```python
from build123d import *

# Parameters (mm, degrees)
SKETCH_1_W                     = 86.9
SKETCH_1_H                     = 86.9
EXTRUDE_1_DEPTH                = 3
HOLE_WIZARD_M2_5_1_D           = 3
HOLE_WIZARD_M2_5_1_DEPTH       = 3
HOLE_WIZARD_M2_5_1_CBORE_D     = 6
HOLE_WIZARD_M2_5_1_CBORE_DEPTH = 2
HOLE_WIZARD_2_0_2_1_D          = 2
HOLE_WIZARD_2_0_2_1_DEPTH      = 3
HOLE_WIZARD_2_5_2_5_1_D        = 2.5
HOLE_WIZARD_2_5_2_5_1_DEPTH    = 3
FILLET_1_R                     = 3
SKETCH_8_R                     = 14
CUT_EXTRUDE_1_DEPTH            = 4


with BuildPart() as part:
    # 草圖1 → 填料-伸長1 (new body)
    with BuildSketch(Plane(origin=(0, -37, 0), x_dir=(1, 0, 0), z_dir=(0, 1, 0))):
        Rectangle(SKETCH_1_W, SKETCH_1_H)
    extrude(amount=-EXTRUDE_1_DEPTH)

    # M2.5 六角頭機械螺釘的柱孔1
    with Locations(Plane(origin=(0, -40, 0), x_dir=(-1, 0, 0), z_dir=(0, -1, 0))):
        with Locations((39, 39), (-39, 39), (-39, -39), (39, -39)):
            CounterBoreHole(HOLE_WIZARD_M2_5_1_D / 2, HOLE_WIZARD_M2_5_1_CBORE_D / 2, HOLE_WIZARD_M2_5_1_CBORE_DEPTH, depth=HOLE_WIZARD_M2_5_1_DEPTH)

    # Ø2.0 (2) 直徑孔1
    with Locations(Plane(origin=(0, -37, 0), x_dir=(1, 0, 0), z_dir=(0, 1, 0))):
        with Locations((5, -10), (0, -10), (-5, -10), (-10, -5), (-10, 0), (-10, 5), (-5, 10), (0, 10), (5, 10), (10, 5), (10, 0), (10, -5), (5, -5), (0, -5), (-5, -5), (-5, 0), (-5, 5), (0, 5), (5, 5), (5, 0), (0, 0), (-37.5, 3), (-37.5, 0), (-37.5, -3), (3, 37.5), (0, 37.5), (-3, 37.5), (37.5, -3), (37.5, 0), (37.5, 3), (-3, -37.5), (0, -37.5), (3, -37.5)):
            Hole(HOLE_WIZARD_2_0_2_1_D / 2, depth=HOLE_WIZARD_2_0_2_1_DEPTH)

    # Ø2.5 (2.5) 直徑孔1
    with Locations(Plane(origin=(0, -40, 0), x_dir=(-1, 0, 0), z_dir=(0, -1, 0))):
        with Locations((12, 12), (-12, 12), (12, -12), (-12, -12)):
            Hole(HOLE_WIZARD_2_5_2_5_1_D / 2, depth=HOLE_WIZARD_2_5_2_5_1_DEPTH)

    # 圓角1
    fillet_1_edges = [part.edges().sort_by_distance(p)[0] for p in [
        (-43.45, -38.5, -43.45),
        (43.45, -38.5, -43.45),
        (43.45, -38.5, 43.45),
        (-43.45, -38.5, 43.45),
    ]]
    fillet(fillet_1_edges, radius=FILLET_1_R)

    # 草圖8 → 除料-伸長1 (cut, through all)
    with BuildSketch(Plane(origin=(0, -37, 0), x_dir=(1, 0, 0), z_dir=(0, 1, 0))):
        Circle(SKETCH_8_R)
        with BuildLine():
            Line((-40.45, -12), (-40.45, 12))
            ThreePointArc((-40.45, 12), (-37.45, 15), (-34.45, 12))
            Line((-34.45, 12), (-34.45, -12))
            ThreePointArc((-34.45, -12), (-37.45, -15), (-40.45, -12))
        make_face()
        with BuildLine():
            Line((-12, 40.45), (12, 40.45))
            ThreePointArc((12, 40.45), (15, 37.45), (12, 34.45))
            Line((12, 34.45), (-12, 34.45))
            ThreePointArc((-12, 34.45), (-15, 37.45), (-12, 40.45))
        make_face()
        with BuildLine():
            Line((40.45, 12), (40.45, -12))
            ThreePointArc((40.45, -12), (37.45, -15), (34.45, -12))
            Line((34.45, -12), (34.45, 12))
            ThreePointArc((34.45, 12), (37.45, 15), (40.45, 12))
        make_face()
        with BuildLine():
            Line((12, -40.45), (-12, -40.45))
            ThreePointArc((-12, -40.45), (-15, -37.45), (-12, -34.45))
            Line((-12, -34.45), (12, -34.45))
            ThreePointArc((12, -34.45), (15, -37.45), (12, -40.45))
        make_face()
    extrude(amount=-CUT_EXTRUDE_1_DEPTH, mode=Mode.SUBTRACT)


solid = part.part
```
Here's how the part is built. I have some questions about the finished solid (model axes, mm). A direction names the side the tool comes from. Coordinates: 2 decimals unless noted, no trailing zeros. Order: outer loops, then holes, each group sorted by start corner. A loop starts at its lowest first (then second) coordinate and runs counter-clockwise, first axis right, second up.
1) Imagine slicing it at B-B on z = 0. List the corners of the cut face in (x, y) for me.
2) We'd pull the mould along Z, two halves only. Please class faces 1 (the face through (42.55, -38.52, -42.59)), 2 (the face through (11.84, -38.48, 10.76)): +Z half, -Z half, draft (parallel to the pull), parting line (faces both ways), or undercut.
3) Imagine slicing it at D-D on z = -9.5. List the corners of the cut face in (x, y) for me, and give its area (3 significant figures).
4) Which directions (+Z, -Z, +X, -X, +Y, -Y) give clear straight access to the entire face, cutting with the end or side of a thin tool? Please do faces 3 (the face through (34.45, -38, 0)), 4 (the face through (-36.79, -39.01, -41.03)), 5 (the face through (-42.59, -38.52, -42.55)).
5) I need wall thicknesses on line 1 (X direction, y = -38.2, z = 0.5); line 2 (Z direction, x = 12, y = -38.8); line 3 (X direction, y = -38.7, z = 14.5). Which ranges of each line are inside material? Lowest first, please.
6) Will this pin go through, and if not, where does the flat tip stop? pin 1 (3.5 mm diameter, centred on x = -39, z = 39, fed in from -Y).
7) Imagine slicing it at A-A on y = -37.45. State how many separate pieces and enclosed holes the cut face has, and give its area (3 significant figures).
8) Imagine slicing it at C-C on x = 39. List the corners of the cut face in (y, z) for me.
Response values:
1. outline: (-43.45, -40) - (-40.45, -40) - (-40.45, -37) - (-43.45, -37) - close; (-34.45, -40) - (-14, -40) - (-14, -37) - (-34.45, -37) - close; (14, -40) - (34.45, -40) - (34.45, -37) - (14, -37) - close; (40.45, -40) - (43.45, -40) - (43.45, -37) - (40.45, -37) - close
2. face 1: -Z half
2. face 2: undercut
3. outline: (-43.45, -40) - (-40.45, -40) - (-40.45, -37) - (-43.45, -37) - close; (-34.45, -40) - (-10.28, -40) - (-10.28, -37) - (-34.45, -37) - close; (10.28, -40) - (34.45, -40) - (34.45, -37) - (10.28, -37) - close; (40.45, -40) - (43.45, -40) - (43.45, -37) - (40.45, -37) - close
3. area: 163 mm2
4. face 3: +Y, -Y
4. face 4: -Y
4. face 5: -Z, -X, +Y, -Y
5. line 1: x = -43.45 to -40.45, -34.45 to -13.99, 13.99 to 34.45, 40.45 to 43.45
5. line 2: z = -43.45 to -40.45, -34.45 to -13.25, -10.75 to -7.21, 7.21 to 10.75, 13.25 to 34.45, 40.45 to 43.45
5. line 3: x = -43.45 to -39.11, -35.79 to 35.79, 39.11 to 43.45
6. pin 1: stops at y = -38
7. separate pieces: 1
7. enclosed holes: 13
7. area: 6,190 mm2
8. outline: (-40, -43.45) - (-37, -43.45) - (-37, -40.5) - (-38, -40.5) - (-38, -42) - (-40, -42) - close; (-40, -36) - (-38, -36) - (-38, -37.5) - (-37, -37.5) - (-37, -14.57) - (-40, -14.57) - close; (-40, 14.57) - (-37, 14.57) - (-37, 37.5) - (-38, 37.5) - (-38, 36) - (-40, 36) - close; (-40, 42) - (-38, 42) - (-38, 40.5) - (-37, 40.5) - (-37, 43.45) - (-40, 43.45) - close
